```python
from build123d import *

# Parameters (mm, degrees)
HOLE_WIZARD_G1_81_D           = 8.8
HOLE_WIZARD_G1_81_DEPTH       = 9
HOLE_WIZARD_G1_81_CSINK_D     = 11.3
HOLE_WIZARD_G1_81_CSINK_ANGLE = 90


with BuildPart() as part:
    # Эскиз2 → Повернуть1 (revolve)
    with BuildSketch(Plane.XY):
        Polygon((-12.8, 2.5), (-12.8, 7.95), (-9.8, 7.95), (-9.8, 6), (-3.7, 6), (-3.7, 7.95), (0, 7.95), (0, 2.5), align=None)
    revolve(axis=Axis((0, 0, 0), (-1, 0, 0)))

    # Отверстие обработанное метчиком G1/81
    with Locations(Plane(origin=(-12.8, 0, 0), x_dir=(0, -1, 0), z_dir=(-1, 0, 0))):
        with Locations((0, 0)):
            CounterSinkHole(HOLE_WIZARD_G1_81_D / 2, HOLE_WIZARD_G1_81_CSINK_D / 2, depth=HOLE_WIZARD_G1_81_DEPTH, counter_sink_angle=HOLE_WIZARD_G1_81_CSINK_ANGLE)


solid = part.part
```
Geometry check sheet. Reference: the model listing, model coordinates, mm. A direction names the side the tool comes from. Round coordinates to 2 decimals unless told otherwise and drop trailing zeros. Order: outer loops, then holes, each group sorted by start corner. A loop starts at its lowest first (then second) coordinate and runs counter-clockwise, first axis right, second up. Notation, with made-up numbers: M -32,34 L -22,34 A24 cw -22,45 Z; hole C -37,9 d5. An arc over 180 degrees is marked long. Write item = value, one per line.
Q1. Scan lines: line 1 (X direction, y = 1, z = 6); line 2 (Z direction, x = -2.9, y = 0); line 3 (Y direction, x = -6, z = 0). Record each from-to range of solid material in increasing order.
Answer block:
line_1 = -12.8 to -9.8, -3.7 to 0
line_2 = -7.95 to -2.5, 2.5 to 7.95
line_3 = -6 to -4.4, 4.4 to 6
Q2. Section check C-C (x = -10.5). Enter the section's corners in (y, z).
Answer block:
outline = C 0,0 d15.9; hole C 0,0 d8.8
Q3. Depth check by flat-ended pin: pin 1 Ø5.5 at (y, z) = (0, 0) entering from -X; pin 2 Ø4 at (y, z) = (0, 0) entering from +X; pin 3 Ø2 at (x, z) = (-4, -2.5) entering from -Y; pin 4 Ø3 at (x, y) = (-5, -2.5) entering from -Z. Enter the tip coordinate at first touch or a pass-through.
Answer block:
pin_1 = -3.8
pin_2 = through
pin_3 = -7.8
pin_4 = -7.75
Q4. Release check for a two-part mould opening along Y. For faces 4 (the flat face through (0, 2, -2)), 5 (the cylindrical face through (-1.93, -0.54, 2.44)), 6 (the cylindrical face through (-1.82, -1.72, 7.76)) record: released by +Y, released by -Y, zero draft, split by the parting line, or undercut.
Answer block:
face_4 = zero draft
face_5 = undercut
face_6 = split by the parting line
Q5. Section check D-D (z = 6.5). Enter the section's corners in (x, y).
Answer block:
outline = M -12.8,-4.58 L -9.8,-4.58 L -9.8,4.58 L -12.8,4.58 Z; M -3.7,-4.58 L 0,-4.58 L 0,4.58 L -3.7,4.58 Z
Q6. Section check A-A (z = 0). Enter the section's corners in (x, y).
Answer block:
outline = M -12.8,-7.95 L -9.8,-7.95 L -9.8,-6 L -3.7,-6 L -3.7,-7.95 L 0,-7.95 L 0,-2.5 L -3.8,-2.5 L -3.8,-4.4 L -11.55,-4.4 L -12.8,-5.65 Z; M -12.8,5.65 L -11.55,4.4 L -3.8,4.4 L -3.8,2.5 L 0,2.5 L 0,7.95 L -3.7,7.95 L -3.7,6 L -9.8,6 L -9.8,7.95 L -12.8,7.95 Z
Q7. Set-up check for faces 1 (the cylindrical face through (-7, -6, 0)), 2 (the cylindrical face through (-7.621, 4.197, 1.322)), 3 (the flat face through (-12.8, -3, 5)): record each of +Z, -Z, +X, -X, +Y, -Y from which the full face is reachable in a straight line by a thin tool's end or side.
Answer block:
face_1 = none
face_2 = -X
face_3 = +Z, -Z, -X, +Y, -Y
